from build123d import *

# Parameters (mm, degrees)
BOSS_EXTRUDE1_DEPTH     = 60
BOSS_EXTRUDE2_DEPTH     = 40
CUT_EXTRUDE1_DEPTH      = 182.107702763
CUT_EXTRUDE1_DEPTH_BACK = 182.107702763


with BuildPart() as part:
    # Sketch1 → Boss-Extrude1 (new, symmetric)
    with BuildSketch(Plane.YZ):
        Polygon((70, 0), (160, 0), (160, 100), (130, 100), (130, 90), (140, 90), (140, 80), (90, 80), (90, 90), (100, 90), (100, 100), (70, 100), align=None)
    extrude(amount=BOSS_EXTRUDE1_DEPTH, both=True)

    # Sketch1_3 → Boss-Extrude2 (add, symmetric)
    with BuildSketch(Plane.YZ):
        Polygon((70, 40), (0, 40), (0, 0), (10, 0), (10, 10), (60, 10), (60, 0), (70, 0), align=None)
    extrude(amount=BOSS_EXTRUDE2_DEPTH, both=True)

    # Sketch2 → Cut-Extrude1 (cut, two sides: drawn at the far end of the back side and taken through both)
    with BuildSketch(Plane.XY.offset(40).offset(-CUT_EXTRUDE1_DEPTH_BACK)):
        with BuildLine():
            Line((-15, 50), (15, 50))
            ThreePointArc((15, 50), (30, 35), (15, 20))
            Line((15, 20), (-15, 20))
            ThreePointArc((-15, 20), (-30, 35), (-15, 50))
        make_face()
    extrude(amount=CUT_EXTRUDE1_DEPTH + CUT_EXTRUDE1_DEPTH_BACK, mode=Mode.SUBTRACT)


solid = part.part
Can you work these out from the model? Positions are in its coordinate system, mm. A direction names the side the tool comes from. Round coordinates to 2 decimals unless told otherwise and drop trailing zeros. Loops run counter-clockwise (first coordinate to the right, second up) from the corner with the lowest first, then second, coordinate; pieces in that order, holes last. Notation, with made-up numbers: (76.5, 71.5) - (130.5, 71.5) arc R19 ccw to (130.5, 78.5) - close; hole circle Ø9 at (-22.75, 51.25). An arc over 180 degrees is marked (long way). Answer in a Markdown table with one row per item. Add a question column.
Q1. Which directions (+Z, -Z, +X, -X, +Y, -Y) give clear straight access to the entire face, cutting with the end or side of a thin tool? Please do faces 5 (the flat face through (1, 130, 95)), 6 (the cylindrical face through (-30, 35, 25)), 7 (the flat face through (1, 51, 40)), 8 (the flat face through (1, 95, 90)).
Q2. We'd pull the mould along Y, two halves only. Please class faces 1 (the flat face through (0, 50, 25)), 2 (the cylindrical face through (30, 35, 25)), 3 (the flat face through (1, 0, 20)), 4 (the flat face through (1, 5, 0)): pulls with the +Y half, pulls with the -Y half, needs draft (parallel to the pull), parting line crosses it, or undercut.
Q3. I want a section at B-B on x = 8.5. List the corners of the cut face in (y, z) for me, and give its area (3 significant figures).
Q4. I want a section at A-A on y = 35. List the corners of the cut face in (x, z) for me, and give its area (3 significant figures).
Q5. I need wall thicknesses on L1, parallel to Z at x = 45.5, y = 95; L2, parallel to Y at x = 5, z = 6; L3, parallel to Y at x = 47, z = 57. Which ranges of each line are inside material? Lowest first, please.
Q6. I want a section at D-D on y = 95. List the corners of the cut face in (x, z) for me.
Q7. For pin 1 Ø11 at (x, z) = (29.5, 83.5) entering from -Y; pin 2 Ø20 at (y, z) = (20, 26) entering from +X; pin 3 Ø15 at (x, y) = (-15.5, 23.5) entering from -Z, each with a flat end and sliding along its axis, tell me the tip position at first contact or that it passes through.
Q8. I want a section at C-C on z = 20. List the corners of the cut face in (x, y) for me.
A:
| question | item | result |
|---|---|---|
| 1 | face 5 | +Z, +X, -X |
| 1 | face 6 | +Z, -Z |
| 1 | face 7 | +Z, +X, -X, -Y |
| 1 | face 8 | +X, -X |
| 2 | face 1 | undercut |
| 2 | face 2 | undercut |
| 2 | face 3 | pulls with the -Y half |
| 2 | face 4 | needs draft |
| 3 | outline | (0, 0) - (10, 0) - (10, 10) - (20, 10) - (20, 40) - (0, 40) - close; (50, 10) - (60, 10) - (60, 0) - (160, 0) - (160, 100) - (130, 100) - (130, 90) - (140, 90) - (140, 80) - (90, 80) - (90, 90) - (100, 90) - (100, 100) - (70, 100) - (70, 40) - (50, 40) - close |
| 3 | area | 9,600 mm^2 |
| 4 | outline | (-40, 10) - (-30, 10) - (-30, 40) - (-40, 40) - close; (30, 10) - (40, 10) - (40, 40) - (30, 40) - close |
| 4 | area | 600 mm^2 |
| 5 | L1 | 0 to 80, 90 to 100 |
| 5 | L2 | 0 to 10, 60 to 160 |
| 5 | L3 | 70 to 160 |
| 6 | outline | (-60, 0) - (60, 0) - (60, 80) - (-60, 80) - close; (-60, 90) - (60, 90) - (60, 100) - (-60, 100) - close |
| 7 | pin 1 | y = 70 |
| 7 | pin 2 | x = 40 |
| 7 | pin 3 | z = 10 |
| 8 | outline | (-60, 70) - (-40, 70) - (-40, 0) - (40, 0) - (40, 70) - (60, 70) - (60, 160) - (-60, 160) - close; hole (-15, 20) - (15, 20) arc R15 ccw to (15, 50) - (-15, 50) arc R15 ccw to start |
